from build123d import *

# Parameters (mm, degrees)
CYLINDER001_R          = 2.1
CYLINDER001_DEPTH      = 30
CYLINDER003_R          = 2.95
CYLINDER003_DEPTH      = 4
CYLINDER002_R          = 1.9
CYLINDER002_DEPTH      = 10
PRISM_DEPTH            = 3
FUSION_ROLL_ANGLE      = -90
FUSION_PITCH_ANGLE     = -60
FUSION_PLACEMENT_ANGLE = 90
CLONE_ROLL_ANGLE       = -3.3e-05
CLONE_PITCH_ANGLE      = -2.6e-05
CLONE_PLACEMENT_ANGLE  = 7e-06
SKETCH001_W            = 2
SKETCH001_H            = 14
PAD001_DEPTH           = 30
CYLINDER_R             = 4.2
CYLINDER_DEPTH         = 30
PAD_DEPTH              = 28


with BuildPart() as top_screw_cut:
    # Cylinder001 → Cylinder001 (new body)
    with BuildSketch(Plane(origin=(-30, 12, -1), x_dir=(1, 0, 0), z_dir=(0, 0, 1))):
        Circle(CYLINDER001_R)
    extrude(amount=CYLINDER001_DEPTH)


with BuildPart() as cylinder001:
    # Cylinder003 → Cylinder003 (new body)
    with BuildSketch(Plane.XY.offset(10)):
        Circle(CYLINDER003_R)
    extrude(amount=CYLINDER003_DEPTH)


with BuildPart() as cylinder:
    # Cylinder002 → Cylinder002 (new body)
    with BuildSketch(Plane.XY):
        Circle(CYLINDER002_R)
    extrude(amount=CYLINDER002_DEPTH)


with BuildPart() as fusion:
    # Prism → Prism (new body)
    with BuildSketch(Plane.XY.offset(-1)):
        Polygon((3.45, 0), (1.725, 2.987788), (-1.725, 2.987788), (-3.45, 0), (-1.725, -2.987788), (1.725, -2.987788), align=None)
    extrude(amount=PRISM_DEPTH)

    # Fusion: union Cylinder001, Cylinder
    add(cylinder001.part)
    add(cylinder.part)


with BuildPart() as fusion_1:
    # Fusion roll: moved
    add(fusion.part.rotate(Axis((0, 0, 0), (1, 0, 0)), FUSION_ROLL_ANGLE))


with BuildPart() as fusion_2:
    # Fusion pitch: moved
    add(fusion_1.part.rotate(Axis((0, 0, 0), (0, 1, 0)), FUSION_PITCH_ANGLE))


with BuildPart() as fusion_3:
    # Fusion placement: moved
    add(fusion_2.part.moved(Location((-24, -6, 7))).rotate(Axis((-24, -6, 7), (0, 0, 1)), FUSION_PLACEMENT_ANGLE))


with BuildPart() as clamps_screw_cut:
    # Clone base: copy of Fusion
    add(fusion_3.part)


with BuildPart() as clamps_screw_cut_1:
    # Clone roll: moved
    add(clamps_screw_cut.part.rotate(Axis((0, 0, 0), (1, 0, 0)), CLONE_ROLL_ANGLE))


with BuildPart() as clamps_screw_cut_2:
    # Clone pitch: moved
    add(clamps_screw_cut_1.part.rotate(Axis((0, 0, 0), (0, 1, 0)), CLONE_PITCH_ANGLE))


with BuildPart() as clamps_screw_cut_3:
    # Clone placement: moved
    add(clamps_screw_cut_2.part.moved(Location((2e-06, -1e-06, 14.000007))).rotate(Axis((2e-06, -1e-06, 14.000007), (0, 0, 1)), CLONE_PLACEMENT_ANGLE))

    # Fusion001: union Fusion
    add(fusion_3.part)


with BuildPart() as clamps_relief_cut:
    # Sketch001 → Pad001 (new body)
    with BuildSketch(Plane.XY.offset(-1)):
        with Locations((-30, -7)):
            Rectangle(SKETCH001_W, SKETCH001_H)
    extrude(amount=PAD001_DEPTH)


with BuildPart() as fusion002:
    # Cylinder → Cylinder (new body)
    with BuildSketch(Plane(origin=(-30, 0, -1), x_dir=(1, 0, 0), z_dir=(0, 0, 1))):
        Circle(CYLINDER_R)
    extrude(amount=CYLINDER_DEPTH)

    # Fusion002: union Top_screw_cut, Clamps_Screw_cut, Clamps_Relief_cut
    add(top_screw_cut.part)
    add(clamps_screw_cut_3.part)
    add(clamps_relief_cut.part)


with BuildPart() as cut:
    # Sketch → Pad (new body)
    with BuildSketch(Plane.XY):
        with BuildLine():
            ThreePointArc((-24, 10), (-30, 16), (-36, 10))
            Line((-36, -12), (-36, 10))
            Line((-24, -12), (-36, -12))
            Line((-24, 5), (-24, -12))
            Line((0, 5), (-24, 5))
            Line((0, 10), (0, 5))
            Line((-24, 10), (0, 10))
        make_face()
    extrude(amount=PAD_DEPTH)

    # Cut: cut Fusion002
    add(fusion002.part, mode=Mode.SUBTRACT)


with BuildPart() as fusion003:
    # Part__Mirroring: instance of Cut
    add(cut.part.mirror(Plane(origin=(0, 0, 0), x_dir=(0, -1, 0), z_dir=(1, 0, 0))))

    # Fusion003: union Cut
    add(cut.part)


solid = fusion003.part
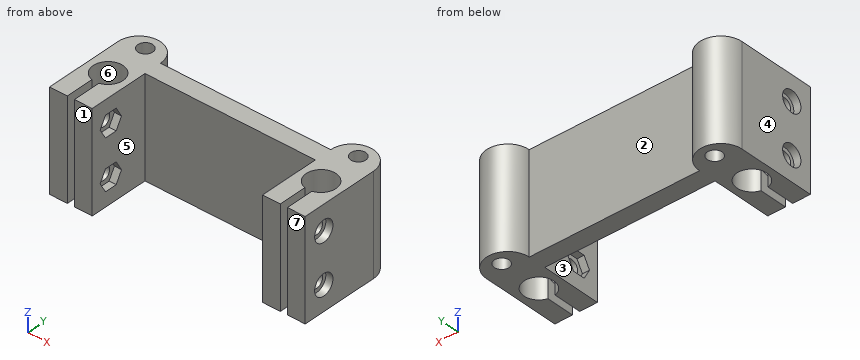
For this review, take the finished solid that the model builds, in its own axes (mm). Face numbers are marked on the shaded views. A direction names the side the tool comes from. Give positions to 0.01 mm unless a question says otherwise; leave off trailing zeros. Order: outer loops, then holes, each group sorted by start corner. A loop starts at its lowest first (then second) coordinate and runs counter-clockwise, first axis right, second up. Notation, with made-up numbers: (73.5, 59) - (105.5, 59) arc R28 ccw to (105.5, 80) - close; hole circle Ø2 at (79.5, 29). An arc over 180 degrees is marked (long way). Answer as a JSON object with one key per item and string values. Group by question number.
Item 1: Wall thickness on line 1 along Z through (x, y) = (33, -6); line 2 along X through (y, z) = (12.75, 13.5); line 3 along X through (y, z) = (13.25, 7.5): over which ranges is each line inside the solid? List them lowest first.
Item 2: Clearance check with flat-ended pins moving along their axes: pin 1 Ø3.5 at (y, z) = (-6, 7) entering from +X; pin 2 Ø5 at (y, z) = (-6, 7) entering from +X; pin 3 Ø1 at (x, z) = (10.5, 22.5) entering from -Y; pin 4 Ø5 at (x, z) = (-14.5, 18.5) entering from +Y. State where each tip first meets the part, or that it passes through.
Item 3: Take a section at A-A on y = -10.5. Give the boundary of the cut face in (x, z).
Item 4: Take a section at B-B on x = 30. Give the boundary of the cut face in (y, z), and give its area (3 significant figures).
Item 5: Take a section at C-C on z = 12.75. Give the boundary of the cut face in (x, y).
Item 6: Draft analysis for pull direction X (two halves, no side actions). For the marked faces 4, 5, 6 and 7, state which applies: pulls with the +X half, pulls with the -X half, needs draft (parallel to the pull), parting line crosses it, or undercut.
Item 7: Machinability: for the marked faces 1, 2 and 3, which of the approach directions +Z, -Z, +X, -X, +Y, -Y give a long, thin tool a straight path to every point of the face, cutting with its end or side? Answer none if there is none.
Item 8: Take a section at D-D on y = -6. Give the number of separate pieces and of enclosed holes in the cut face, and give its area (3 significant figures).
Reported:
{
 "1": {"line 1": "0 to 5.1, 8.9 to 19.1, 22.9 to 28", "line 2": "-35.33 to -31.96, -28.04 to -24.67, 24.67 to 28.04, 31.96 to 35.33", "line 3": "-35.04 to -31.69, -28.31 to -24.96, 24.96 to 28.31, 31.69 to 35.04"},
 "2": {"pin 1": "through", "pin 2": "x = 34", "pin 3": "y = 5", "pin 4": "y = 10"},
 "3": {"outline": "(-36, 0) - (-31, 0) - (-31, 28) - (-36, 28) - close; (-29, 0) - (-24, 0) - (-24, 28) - (-29, 28) - close; (24, 0) - (29, 0) - (29, 28) - (24, 28) - close; (31, 0) - (36, 0) - (36, 28) - (31, 28) - close"},
 "4": {"outline": "(4.2, 0) - (9.9, 0) - (9.9, 28) - (4.2, 28) - close; (14.1, 0) - (16, 0) - (16, 28) - (14.1, 28) - close", "area": "213 mm^2"},
 "5": {"outline": "(-36, -12) - (-31, -12) - (-31, -4.08) arc R4.2 cw (long way) to (-29, -4.08) - (-29, -12) - (-24, -12) - (-24, 5) - (24, 5) - (24, -12) - (29, -12) - (29, -4.08) arc R4.2 cw (long way) to (31, -4.08) - (31, -12) - (36, -12) - (36, 10) arc R6 ccw to (24, 10) - (-24, 10) arc R6 ccw to (-36, 10) - close; hole circle Ø4.2 at (-30, 12); hole circle Ø4.2 at (30, 12)"},
 "6": {"face 4": "pulls with the -X half", "face 5": "undercut", "face 6": "undercut", "face 7": "needs draft"},
 "7": {"face 1": "+Z, -Z, +X, -X, -Y", "face 2": "+Z, -Z, +Y", "face 3": "+Z, -Z, -Y"},
 "8": {"separate pieces": "12", "enclosed holes": "0", "area": "374 mm^2"}
}
